Design review of the part built by this model. Coordinates are the model's own, in mm. Round coordinates to 2 decimals unless told otherwise and drop trailing zeros. Write each loop counter-clockwise with the first axis right and the second up, starting at its lowest first coordinate (ties: lowest second). Pieces come first, ordered by that corner, then holes. Notation, with made-up numbers: (-30.5, -28.5) - (2.5, -28.5) arc R26 ccw to (2.5, -9.5) - close; hole circle Ø2 at (3.5, -4.75). An arc over 180 degrees is marked (long way). Use one line per item in the form item = value.
Autodesk Inventor part; units mm, degrees
ref_plane "YZ Plane" through (0, 0, 0) normal (1, 0, 0) x (0, 1, 0)
ref_plane "XZ Plane" through (0, 0, 0) normal (0, 1, 0) x (-1, 0, 0)
ref_plane "XY Plane" through (0, 0, 0) normal (0, 0, 1) x (1, 0, 0)
sketch "Sketch2" plane through (0, 0, 0) normal (0, 0, 1) x (1, 0, 0)
  line L0 (1.55, 6.5) -> (-1.55, 6.5)
  line L1 (-1.55, 6.5) -> (-1.55, 5.3)
  line L2 (-1.55, 5.3) -> (1.55, 5.3)
  line L3 (1.55, 5.3) -> (1.55, 6.5)
  arc A0 (0.8944, 5.3) -> (-0.8944, 5.3) centre (0, 4.5) ccw
  line L4 (-2.17, 0) -> (2.17, 0)
  point P0 (0, 0)
  dimension "d8" = 3.1
  dimension "d9" = 1.2
  dimension "d10" = 1.55
  dimension "d11" = 5.3
  dimension "d12" = 0.8
  dimension "d13" = 1.2
revolve "Revolution2" add sketch "Sketch2" angle 360 about axis through (-10, 0, 0) along (1, 0, 0) contours L3 L2 A0 L1 L0
fillet "Fillet1" radius 0.21 2 edges at (1.55, -6.5, 0) (-1.55, -6.5, 0)
properties part number "Outer Ring(fixed)"
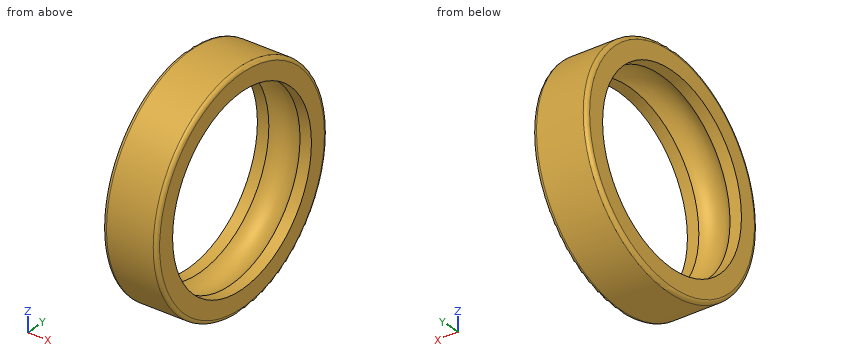
Q1. To check wall thickness, follow line 1 along Y through (x, z) = (-0.3, -0.25); line 2 along Z through (x, y) = (-0.3, -4.5); line 3 along Y through (x, z) = (-0.75, -3.75). State the ranges of each line that lie inside material, in increasing order. Write a range as from..to.
Calculated:
line_1 = -6.5..-5.66, 5.66..6.5
line_2 = -4.69..-3.44, 3.44..4.69
line_3 = -5.31..-3.94, 3.94..5.31
Q2. For P1, Ø3, axis at y = 1.5, z = 1, coming from the -X side; P2, Ø5, axis at y = 1.5, z = -4.5, coming from the -X side; P3, Ø1, axis at x = 0, y = 2, coming from the -Z side, all flat-tipped, find the tip position at first contact; note any pin that passes through.
Calculated:
P1 = through
P2 = -1.55
P3 = -6.32
Q3. We need section C-C on x = 1.15. Write out the cut boundary in (y, z), then the cut area to 3 significant figures.
Calculated:
outline = circle Ø13 at (0, 0); hole circle Ø10.6 at (0, 0)
area = 44.5 mm2
Q4. We need section A-A on z = 0. Write out the cut boundary in (x, y), then the cut area to 3 significant figures.
Calculated:
outline = (-1.55, -6.29) arc R0.21 ccw to (-1.34, -6.5) - (1.34, -6.5) arc R0.21 ccw to (1.55, -6.29) - (1.55, -5.3) - (0.89, -5.3) arc R1.2 cw to (-0.89, -5.3) - (-1.55, -5.3) - close; (-1.55, 5.3) - (-0.89, 5.3) arc R1.2 cw to (0.89, 5.3) - (1.55, 5.3) - (1.55, 6.29) arc R0.21 ccw to (1.34, 6.5) - (-1.34, 6.5) arc R0.21 ccw to (-1.55, 6.29) - close
area = 6.41 mm2
Q5. We need section D-D on x = -0.35. Write out the cut boundary in (y, z).
Calculated:
outline = circle Ø13 at (0, 0); hole circle Ø11.3 at (0, 0)
